Could you check a few things on this drawing? It's one solid part, dimensions in mm from its lowest x, y, z. A direction names the side the tool comes from. Give positions to 0.01 mm unless a question says otherwise; leave off trailing zeros. Order: outer loops, then holes, each group sorted by start corner. A loop starts at its lowest first (then second) coordinate and runs counter-clockwise, first axis right, second up.
Item 1: I want a section at C-C, the plane y = 8. Write out the boundary of the cut face in (x, z).
Item 2: I want a section at A-A, the plane x = 21. Write out the boundary of the cut face in (y, z), then the cut area to 3 significant figures.
Item 3: I want a section at B-B, the plane y = 23.5. Write out the boundary of the cut face in (x, z), then the cut area to 3 significant figures.
Item 4: I want a section at D-D, the plane z = 11. Write out the boundary of the cut face in (x, y), then the cut area to 3 significant figures.
Item 5: I'm going to push flat-ended pins straight in: pin 1 Ø12 at (x, y) = (30, 31.5) entering from -Z; pin 2 Ø5 at (x, z) = (35, 15) entering from -Y; pin 3 Ø3 at (x, z) = (6, 26) entering from +Y; pin 4 Ø1.5 at (x, y) = (21.5, 34.5) entering from +Z. Where does each tip first touch, or does it pass through?
Item 6: Which directions (+Z, -Z, +X, -X, +Y, -Y) give clear straight access to the entire face, cutting with the end or side of a thin tool? Please do the marked faces 1 and 2.
Item 7: If I drill on line 1 along Y through (x, z) = (5, 32); line 2 along Y through (x, z) = (21, 32); line 3 along Y through (x, z) = (33, 8.5), over which ranges is the centre line in solid material (lowest first)?
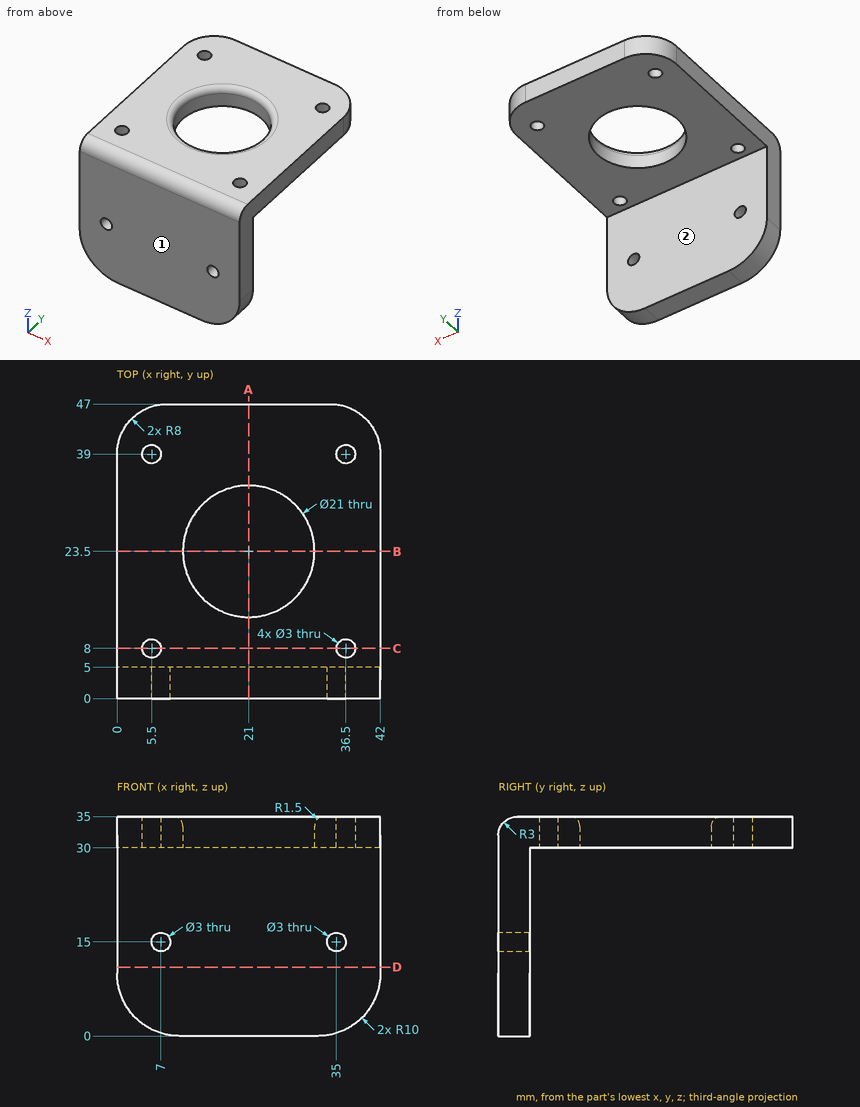
Results list:
1. outline: (0, 30) - (4, 30) - (4, 35) - (0, 35) - close; (7, 30) - (35, 30) - (35, 35) - (7, 35) - close; (38, 30) - (42, 30) - (42, 35) - (38, 35) - close
2. outline: (0, 0) - (5, 0) - (5, 30) - (13, 30) - (13, 33.5) arc R1.5 ccw to (11.5, 35) - (3, 35) arc R3 ccw to (0, 32) - close; (34, 30) - (47, 30) - (47, 35) - (35.5, 35) arc R1.5 ccw to (34, 33.5) - close
2. area: 277 mm2
3. outline: (0, 30) - (10.5, 30) - (10.5, 33.5) arc R1.5 ccw to (9, 35) - (0, 35) - close; (31.5, 30) - (42, 30) - (42, 35) - (33, 35) arc R1.5 ccw to (31.5, 33.5) - close
3. area: 104 mm2
4. outline: (0, 0) - (42, 0) - (42, 5) - (0, 5) - close
4. area: 210 mm2
5. pin 1: stops at z = 30
5. pin 2: stops at y = 0
5. pin 3: stops at y = 5
5. pin 4: stops at z = 34.98
6. face 1: +Z, -Z, +X, -X, -Y
6. face 2: -Z, +X, -X, +Y
7. line 1: y = 0 to 6.59, 9.41 to 37.59, 40.41 to 46.42
7. line 2: y = 0 to 13, 34 to 47
7. line 3: y = 0 to 5
